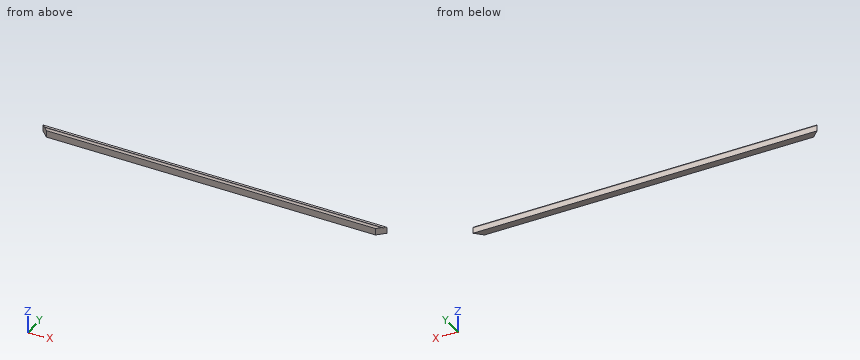
from build123d import *

# Parameters (mm, degrees)
F1_DEPTH = 736.6
F2_SIZE  = 31.74999


# Not quite as in the source:
# - a fillet or chamfer is up to 0.001 mm smaller than in the source, because OpenCascade refuses the exact size


with BuildPart() as f1:
    # F0 (on Right) → F1 (new body, symmetric)
    with BuildSketch(Plane.YZ):
        with BuildLine():
            Line((-15.875, -14.2875), (15.875, -14.2875))
            Line((15.875, -14.2875), (15.875, 9.525))
            ThreePointArc((15.875, 9.525), (12.4385421004, 14.0991686237), (7.08843051, 12.07220847))
            ThreePointArc((7.08843051, 12.07220847), (5.9853917743, 11.4055483551), (4.789455264, 11.886033552))
            ThreePointArc((4.789455264, 11.886033552), (2.3755826554, 13.6595328458), (-0.5531949, 14.2875))
            Line((-0.5531949, 14.2875), (-15.875, 14.2875))
            Line((-15.875, 14.2875), (-15.875, -14.2875))
        make_face()
    extrude(amount=F1_DEPTH, both=True)

    # F2 (size 31.75 in the source; OpenCascade refuses exactly that, so slightly less here)
    f2_edges = [f1.edges().sort_by_distance(p)[0] for p in [
        (-736.6, -15.875, 0),
        (736.6, -15.875, 0),
    ]]
    chamfer(f2_edges, length=F2_SIZE)


solid = f1.part
For this review, take the finished solid that the model builds, in its own axes (mm). Coordinates: 2 decimals unless noted, no trailing zeros. Order: outer loops, then holes, each group sorted by start corner. A loop starts at its lowest first (then second) coordinate and runs counter-clockwise, first axis right, second up. Notation, with made-up numbers: (6.25, 50) - (36.25, 50) arc R28 ccw to (36.25, 71) - close; hole circle Ø8 at (13, -25.5). An arc over 180 degrees is marked (long way). Use one line per item in the form item = value.
Q1. Consider section C-C (y = -8). Give the boundary of the cut face in (x, z) (1 decimal), then the cut area to 3 significant figures.
Checked values:
outline = (-712.7, -14.3) - (712.7, -14.3) - (712.7, 14.3) - (-712.7, 14.3) - close
area = 40,700 mm2
Q2. For P1, Ø1, axis at y = 9.5, z = 0.5, coming from the -X side (3 decimals); P2, Ø3, axis at y = 1.5, z = 2, coming from the +X side (3 decimals); P3, Ø8, axis at y = 1.5, z = -10.5, coming from the -X side (3 decimals), all flat-tipped, find the tip position at first contact; note any pin that passes through.
Checked values:
P1 = -730.725
P2 = 723.725
P3 = -726.225
Q3. Consider section A-A (x = -4). Give the boundary of the cut face in (y, z) (1 decimal).
Checked values:
outline = (-15.9, -14.3) - (15.9, -14.3) - (15.9, 9.5) arc R4.8 ccw to (7.1, 12.1) arc R1.4 cw to (4.8, 11.9) arc R7.1 ccw to (-0.6, 14.3) - (-15.9, 14.3) - close
Q4. For probe 1 along X at (y, z) = (7, -12.5); probe 2 along Y at (x, z) = (157, 10.5) (3 decimals); probe 3 along X at (y, z) = (5, 11), list the stretches that pass through material, from the lowest coordinate up. Write a range as from..to.
Checked values:
probe_1 = -727.73..727.73
probe_2 = -15.875..15.774
probe_3 = -725.73..725.73
